Source: CAD feature listing. Evaluate the final solid. Frame: model axes, mm. Face numbers are marked on the shaded views. Round coordinates to 2 decimals unless told otherwise and drop trailing zeros. Loops run counter-clockwise (first coordinate to the right, second up) from the corner with the lowest first, then second, coordinate; pieces in that order, holes last. Notation, with made-up numbers: M 1.25,50 L 10.25,50 A15 ccw 10.25,71 Z; hole C -8.5,-19.5 d10. An arc over 180 degrees is marked long. Write each question's results on one line, items separated by ' | '. Start each with the question number.
1. Section A-A on z = 56. Output: boundary loops of the cut face in (x, y).
2. Draft query along Y for the marked faces 1 and 2. Return one class per face: released by +Y, released by -Y, zero draft, split by the parting line, or undercut.
3. Ray query, line 1 (X direction, y = 104.25, z = 75.5); line 2 (Z direction, x = 58, y = 104); line 3 (Z direction, x = 108.5, y = 107.5). Return the intervals inside material, ascending.
4. Contact query for flat-ended pins moving along their axis: pin 1 Ø1.5 at (x, z) = (25.5, 92) entering from -Y; pin 2 Ø3.5 at (x, y) = (64, 106) entering from -Z; pin 3 Ø0.9 at (y, z) = (106, 82.5) entering from -X. Output: stop coordinate, or through.
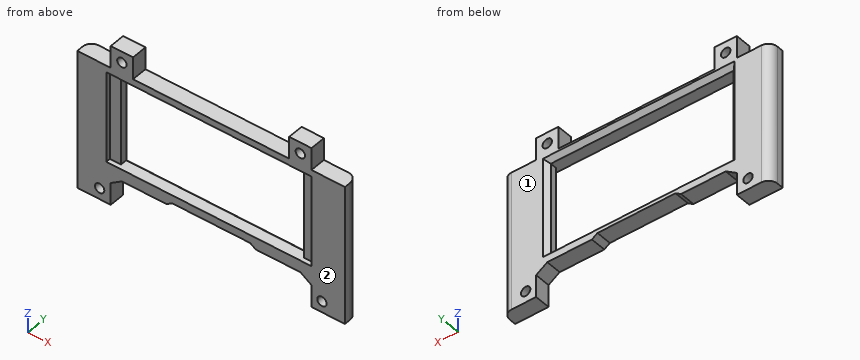
from build123d import *

# Parameters (mm, degrees)
SKETCH_1_R      = 2.1
SKETCH_1_W      = 92
SKETCH_1_H      = 41
EXTRUDE_2_DEPTH = 2
SKETCH_2_R      = 2.1
SKETCH_2_W      = 82.013427323
SKETCH_2_H      = 41
EXTRUDE_5_DEPTH = 5
CHAMFER_START   = 102.001425994
CHAMFER_1_DEPTH = 7
FILLET_1_R      = 4


with BuildPart() as part:
    # Эскиз1 → Бобышка-Вытянуть2 (new body)
    with BuildSketch(Plane(origin=(68.741769048, 102.001425994, 80.052702475), x_dir=(1, 0, 0), z_dir=(0, 1, 0))):
        Polygon((-60, -30), (-45, -30), (-45, -40), (-35, -40), (-35, -30), (35, -30), (35, -40), (45, -40), (45, -30), (60, -30), (60, 32.652702475), (45, 32.652702475), (45, 22.652702475), (55, 22.652702475), (55, 16), (-55, 16), (-55, 22.652702475), (-45, 22.652702475), (-45, 32.652702475), (-60, 32.652702475), align=None)
        with Locations(Location((-50, 27.652702475, 0), (0, 0, 180))):
            Circle(SKETCH_1_R, mode=Mode.SUBTRACT)
        with Locations(Location((49.694344906, 27.652702475, 0), (0, 0, 180))):
            Circle(SKETCH_1_R, mode=Mode.SUBTRACT)
        with Locations(Location((40, -35, 0), (0, 0, 180))):
            Circle(SKETCH_1_R, mode=Mode.SUBTRACT)
        with Locations(Location((-40, -35, 0), (0, 0, 180))):
            Circle(SKETCH_1_R, mode=Mode.SUBTRACT)
        with Locations((-1, -6.5)):
            Rectangle(SKETCH_1_W, SKETCH_1_H, mode=Mode.SUBTRACT)
    extrude(amount=EXTRUDE_2_DEPTH)

    # Эскиз2 → Бобышка-Вытянуть5 (add)
    with BuildSketch(Plane(origin=(0, 104.001425994, 0), x_dir=(1, 0, 0), z_dir=(0, 1, 0))):
        Polygon((23.741769048, -57.4), (23.741769048, -47.4), (8.741769048, -47.4), (8.741769048, -110.052702475), (23.741769048, -110.052702475), (23.741769048, -120.052702475), (33.741769048, -120.052702475), (33.741769048, -110.052702475), (103.741769048, -110.052702475), (103.741769048, -120.052702475), (113.741769048, -120.052702475), (113.741769048, -110.052702475), (128.741769048, -110.052702475), (128.741769048, -47.4), (113.741769048, -47.4), (113.741769048, -57.4), (123.741769048, -57.4), (123.741769048, -64.052702475), (13.741769048, -64.052702475), (13.741769048, -57.4), align=None)
        with Locations(Location((18.741769048, -52.4, 0), (0, 0, 180))):
            Circle(SKETCH_2_R, mode=Mode.SUBTRACT)
        with Locations(Location((118.436113954, -52.4, 0), (0, 0, 180))):
            Circle(SKETCH_2_R, mode=Mode.SUBTRACT)
        with Locations(Location((108.741769048, -115.052702475, 0), (0, 0, 180))):
            Circle(SKETCH_2_R, mode=Mode.SUBTRACT)
        with Locations(Location((28.741769048, -115.052702475, 0), (0, 0, 180))):
            Circle(SKETCH_2_R, mode=Mode.SUBTRACT)
        with Locations((67.735055387, -86.552702475)):
            Rectangle(SKETCH_2_W, SKETCH_2_H, mode=Mode.SUBTRACT)
    extrude(amount=EXTRUDE_5_DEPTH)

    # Фаска1: read off the stored shape, not the designer's step
    # Фаска1 outline → Фаска1 (add)
    with BuildSketch(Plane(origin=(0, 0, 0), x_dir=(1, 0, 0), z_dir=(0, 1, 0)).offset(CHAMFER_START)):
        Polygon((28.741769048, -60.726351237), (23.741769048, -57.4), (13.741769048, -57.4), (13.741769048, -64.052702475), (123.741769048, -64.052702475), (123.741769048, -57.4), (113.741769048, -57.4), (108.741769048, -60.726351237), (88.741769048, -60.726351237), (86.241769048, -62.389526856), (51.241769048, -62.389526856), (48.741769048, -60.726351237), align=None)
    extrude(amount=CHAMFER_1_DEPTH)

    # Chamfer 1 2: loft between two sections, ruled curve by curve
    chamfer_1_2_from = [
        Edge.make_line((26.728341725, 107.001425994, 66.052702475), (26.728341725, 107.001425994, 107.052702475)),
        Edge.make_line((26.728341725, 107.001425994, 107.052702475), (108.741769048, 107.001425994, 107.052702475)),
        Edge.make_line((26.728341725, 107.001425994, 66.052702475), (108.741769048, 107.001425994, 66.052702475)),
        Edge.make_line((108.741769048, 107.001425994, 107.052702475), (108.741769048, 107.001425994, 66.052702475)),
    ]
    chamfer_1_2_to = [
        Edge.make_line((24.728341725, 109.001425994, 64.052702475), (24.728341725, 109.001425994, 109.052702475)),
        Edge.make_line((24.728341725, 109.001425994, 109.052702475), (110.741769048, 109.001425994, 109.052702475)),
        Edge.make_line((24.728341725, 109.001425994, 64.052702475), (110.741769048, 109.001425994, 64.052702475)),
        Edge.make_line((110.741769048, 109.001425994, 109.052702475), (110.741769048, 109.001425994, 64.052702475)),
    ]
    chamfer_1_2 = Solid(Shell([*[Face.make_surface_from_curves(chamfer_1_2_from[k], chamfer_1_2_to[k]) for k in range(4)], Face(Wire(chamfer_1_2_from)), Face(Wire(chamfer_1_2_to))]))
    add(chamfer_1_2, mode=Mode.SUBTRACT)

    # Скругление1
    fillet_1_edges = [part.edges().sort_by_distance(p)[0] for p in [
        (8.741769048, 109.001425994, 78.726351237),
        (128.741769048, 109.001425994, 78.726351237),
    ]]
    fillet(fillet_1_edges, radius=FILLET_1_R)


solid = part.part
Taken from the geometry:
1) outline: M 8.74,102 L 23.74,102 L 23.74,109 L 12.74,109 A4 ccw 8.74,105 Z; M 113.74,102 L 128.74,102 L 128.74,105 A4 ccw 124.74,109 L 113.74,109 Z
2) face 1: released by +Y | face 2: released by -Y
3) line 1: 8.74 to 26.73, 108.74 to 128.74 | line 2: 62.39 to 66.05, 107.05 to 110.05 | line 3: 60.73 to 65.55, 107.55 to 112.97, 117.14 to 120.05
4) pin 1: y = 104 | pin 2: z = 62.39 | pin 3: x = 8.78
